```python
from build123d import *

# Parameters (mm, degrees)
BOSS_EXTRUDE1_DEPTH       = 3.5
SKETCH2_R                 = 9.5
CUT_EXTRUDE1_DEPTH        = 5
SKETCH3_R                 = 8.75
CUT_EXTRUDE2_DEPTH        = 59.736700622
SKETCH4_R                 = 9.5
CUT_EXTRUDE3_DEPTH        = 5
SKETCH5_R                 = 8.75
CUT_EXTRUDE4_DEPTH        = 59.736700622
SKETCH6_R                 = 17.5
SKETCH6_R_2               = 10
CUT_EXTRUDE5_DEPTH        = 0.5
SKETCH7_W                 = 1.5
SKETCH7_H                 = 1.5
FILLET1_START             = 2
FILLET1_DEPTH             = 2
MIRROR2_COPY_1_SKETCH_R   = 17.5
MIRROR2_COPY_1_SKETCH_R_2 = 10
MIRROR2_COPY_1_DEPTH      = 0.5
MIRROR2_COPY_2_SKETCH_W   = 1.5
MIRROR2_COPY_2_SKETCH_H   = 1.5
MIRROR2_START             = 2
MIRROR2_COPY_3_DEPTH      = 2


with BuildPart() as part:
    # Sketch1 → Boss-Extrude1 (new, symmetric)
    with BuildSketch(Plane(origin=(0, 0, 0), x_dir=(1, 0, 0), z_dir=(0, 1, 0))):
        with BuildLine():
            ThreePointArc((-21, 14.282856857), (-55, 0), (-21, -14.282856857))
            ThreePointArc((-21, -14.282856857), (0, -5.707142143), (21, -14.282856857))
            ThreePointArc((21, -14.282856857), (55, 0), (21, 14.282856857))
            ThreePointArc((21, 14.282856857), (0, 5.707142143), (-21, 14.282856857))
        make_face()
    extrude(amount=BOSS_EXTRUDE1_DEPTH, both=True)

    # Sketch2 → Cut-Extrude1 (cut)
    with BuildSketch(Plane(origin=(0, 3.5, 0), x_dir=(1, 0, 0), z_dir=(0, 1, 0))):
        with Locations(Location((-35, 0, 0), (0, 0, 270))):
            Circle(SKETCH2_R)
    extrude(amount=-CUT_EXTRUDE1_DEPTH, mode=Mode.SUBTRACT)

    # Sketch3 → Cut-Extrude2 (cut, through all)
    with BuildSketch(Plane(origin=(0, -1.5, 0), x_dir=(1, 0, 0), z_dir=(0, 1, 0))):
        with Locations(Location((-35, 0, 0), (0, 0, 270))):
            Circle(SKETCH3_R)
    extrude(amount=-CUT_EXTRUDE2_DEPTH, mode=Mode.SUBTRACT)

    # Sketch4 → Cut-Extrude3 (cut)
    with BuildSketch(Plane.XZ.offset(3.5)):
        with Locations(Location((35, 0, 0), (0, 0, 270))):
            Circle(SKETCH4_R)
    extrude(amount=-CUT_EXTRUDE3_DEPTH, mode=Mode.SUBTRACT)

    # Sketch5 → Cut-Extrude4 (cut, through all)
    with BuildSketch(Plane.XZ.offset(-1.5)):
        with Locations(Location((35, 0, 0), (0, 0, 270))):
            Circle(SKETCH5_R)
    extrude(amount=-CUT_EXTRUDE4_DEPTH, mode=Mode.SUBTRACT)

    # Sketch6 → Cut-Extrude5 (cut)
    with BuildSketch(Plane(origin=(0, 3.5, 0), x_dir=(1, 0, 0), z_dir=(0, 1, 0))):
        with Locations(Location((-35, 0, 0), (0, 0, 270))):
            Circle(SKETCH6_R)
        with Locations(Location((-35, 0, 0), (0, 0, 270))):
            Circle(SKETCH6_R_2, mode=Mode.SUBTRACT)
    cut_extrude5 = extrude(amount=-CUT_EXTRUDE5_DEPTH, mode=Mode.SUBTRACT)

    # Sketch7 → Cut-Revolve1 (revolve, cut)
    with BuildSketch(Plane.XY, mode=Mode.PRIVATE) as cut_revolve1_sk:
        with Locations((-54.25, 2.75)):
            Rectangle(SKETCH7_W, SKETCH7_H)
    cut_revolve1 = revolve(cut_revolve1_sk.sketch.rotate(Axis((-35, -6.63312042, 0), (0, 1, 0)), 270), axis=Axis((-35, -6.63312042, 0), (0, 1, 0)), mode=Mode.SUBTRACT)

    # Fillet1: read off the stored shape, not the designer's step
    # Fillet1 outline → Fillet1 (cut)
    with BuildSketch(Plane(origin=(0, 0, 0), x_dir=(1, 0, 0), z_dir=(0, 1, 0)).offset(FILLET1_START)):
        with BuildLine():
            ThreePointArc((-21, -14.282856857), (-17.348361604, -11.231963907), (-13.260269064, -8.796823223))
            ThreePointArc((-13.260269064, -8.796823223), (-15.460727643, -8.508452663), (-16.04026091, -6.366183602))
            ThreePointArc((-16.04026091, -6.366183602), (-18.051415131, -10.618167023), (-21, -14.282856857))
        make_face()
        with BuildLine():
            ThreePointArc((-21, 14.282856857), (-18.051415131, 10.618167023), (-16.04026091, 6.366183602))
            ThreePointArc((-16.04026091, 6.366183602), (-15.460727643, 8.508452663), (-13.260269064, 8.796823223))
            ThreePointArc((-13.260269064, 8.796823223), (-17.348361604, 11.231963907), (-21, 14.282856857))
        make_face()
    fillet1 = extrude(amount=FILLET1_DEPTH, mode=Mode.SUBTRACT)

    # Mirror1: Cut-Extrude5, Cut-Revolve1, Fillet1 across plane
    add(cut_extrude5.mirror(Plane.ZX), mode=Mode.SUBTRACT)
    add(cut_revolve1.mirror(Plane.ZX), mode=Mode.SUBTRACT)
    add(fillet1.mirror(Plane.ZX), mode=Mode.SUBTRACT)

    # Mirror2: Cut-Extrude5, Cut-Revolve1, Fillet1 across plane
    add(cut_extrude5.mirror(Plane(origin=(0, 0, 0), x_dir=(0, 0, 1), z_dir=(1, 0, 0))), mode=Mode.SUBTRACT)
    add(cut_revolve1.mirror(Plane(origin=(0, 0, 0), x_dir=(0, 0, 1), z_dir=(1, 0, 0))), mode=Mode.SUBTRACT)
    add(fillet1.mirror(Plane(origin=(0, 0, 0), x_dir=(0, 0, 1), z_dir=(1, 0, 0))), mode=Mode.SUBTRACT)

    # Mirror2 copy 1 sketch → Mirror2 copy 1 (cut)
    with BuildSketch(Plane(origin=(0, -3.5, 0), x_dir=(-1, 0, 0), z_dir=(0, -1, 0))):
        with Locations(Location((-35, 0, 0), (0, 0, 270))):
            Circle(MIRROR2_COPY_1_SKETCH_R)
        with Locations(Location((-35, 0, 0), (0, 0, 270))):
            Circle(MIRROR2_COPY_1_SKETCH_R_2, mode=Mode.SUBTRACT)
    extrude(amount=-MIRROR2_COPY_1_DEPTH, mode=Mode.SUBTRACT)

    # Mirror2 copy 2 sketch → Mirror2 copy 2 (revolve, cut)
    with BuildSketch(Plane(origin=(0, 0, 0), x_dir=(-1, 0, 0), z_dir=(0, 0, 1))):
        with Locations((-54.25, 2.75)):
            Rectangle(MIRROR2_COPY_2_SKETCH_W, MIRROR2_COPY_2_SKETCH_H)
    revolve(axis=Axis((35, 6.63312042, 0), (0, -1, 0)), mode=Mode.SUBTRACT)

    # Mirror2 copy 3 sketch → Mirror2 copy 3 (cut)
    with BuildSketch(Plane(origin=(0, 0, 0), x_dir=(-1, 0, 0), z_dir=(0, -1, 0)).offset(MIRROR2_START)):
        with BuildLine():
            ThreePointArc((-21, -14.282856857), (-17.348361604, -11.231963907), (-13.260269064, -8.796823223))
            ThreePointArc((-13.260269064, -8.796823223), (-15.460727643, -8.508452663), (-16.04026091, -6.366183602))
            ThreePointArc((-16.04026091, -6.366183602), (-18.051415131, -10.618167023), (-21, -14.282856857))
        make_face()
        with BuildLine():
            ThreePointArc((-21, 14.282856857), (-18.051415131, 10.618167023), (-16.04026091, 6.366183602))
            ThreePointArc((-16.04026091, 6.366183602), (-15.460727643, 8.508452663), (-13.260269064, 8.796823223))
            ThreePointArc((-13.260269064, 8.796823223), (-17.348361604, 11.231963907), (-21, 14.282856857))
        make_face()
    extrude(amount=MIRROR2_COPY_3_DEPTH, mode=Mode.SUBTRACT)


solid = part.part
```
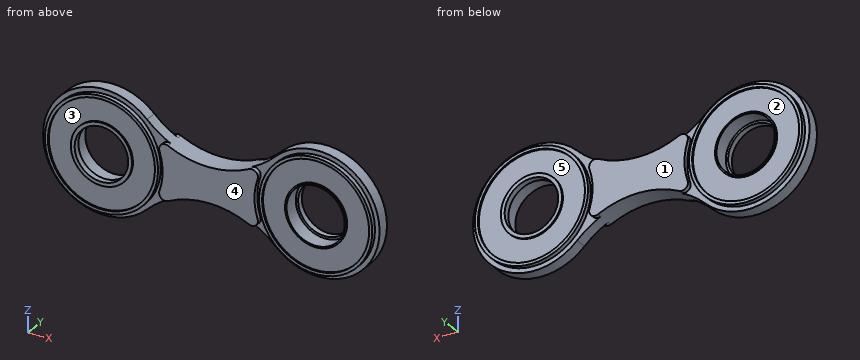
Design review of the part built by this model. Coordinates are the model's own, in mm. Face numbers are marked on the shaded views. A direction names the side the tool comes from. Give positions to 0.01 mm unless a question says otherwise; leave off trailing zeros. Write each loop counter-clockwise with the first axis right and the second up, starting at its lowest first coordinate (ties: lowest second). Pieces come first, ordered by that corner, then holes. Notation, with made-up numbers: (72, -10.5) - (79, -10.5) arc R27 ccw to (79, 7.5) - close; hole circle Ø11 at (40, 11). An arc over 180 degrees is marked (long way). Return JSON: item names as keys, results as strings. Group by question number.
(1) We need section D-D, the plane x = -5.5. Give the boundary of the cut face in (y, z).
(2) We need section A-A, the plane y = 0.25. Give the boundary of the cut face in (x, z), then the cut area to 3 significant figures.
(3) To check wall thickness, follow probe 1 along X at (y, z) = (-0.5, 0.5); probe 2 along X at (y, z) = (-1, 1); probe 3 along X at (y, z) = (-0.75, 8). State the ranges of each line that lie inside material, in increasing order.
(4) We need section C-C, the plane x = -46.5. Give the boundary of the cut face in (y, z), then the cut area to 3 significant figures.
(5) We need section B-B, the plane z = 0. Give the number of separate pieces and of enclosed holes in the cut face, then the cut area to 3 significant figures.
(6) Insertion check: pin 1 (4 mm diameter, centred on x = -20, z = -15, fed in from -Y); pin 2 (1 mm diameter, centred on y = 1, z = -11, fed in from -X); pin 3 (11.5 mm diameter, centred on x = 35, z = 0, fed in from -Y); pin 4 (3 mm diameter, centred on x = -39.5, z = 14.5, fed in from -Y). Each pin has a flat end and moves straight along its axis. Give the tip position at first contact, or say it passes through.
(7) Machinability: for the marked faces 1, 2 and 3, which of the approach directions +Z, -Z, +X, -X, +Y, -Y give a long, thin tool a straight path to every point of the face, cutting with its end or side? Answer none if there is none.
(8) Mouldability with a two-part tool opening along Z and no side actions: class the marked faces 4 and 5 as +Z half, -Z half, draft (parallel to the pull), parting line (faces both ways), or undercut.
Reported:
{
 "1": {"outline": "(-3.5, -6.22) - (3.5, -6.22) - (3.5, 6.22) - (-3.5, 6.22) - close"},
 "2": {"outline": "(-21, -14.28) arc R30 cw to (21, -14.28) arc R20 ccw (long way) to (21, 14.28) arc R30 cw to (-21, 14.28) arc R20 ccw (long way) to start; hole circle Ø19 at (-35, 0); hole circle Ø19 at (35, 0)", "area": "2,410 mm2"},
 "3": {"probe 1": "x = -54.99 to -44.49, -25.51 to 25.51, 44.49 to 54.99", "probe 2": "x = -54.97 to -44.45, -25.55 to 25.55, 44.45 to 54.97", "probe 3": "x = -53.33 to -40.12, -29.88 to -11.5, 11.5 to 29.88, 40.12 to 53.33"},
 "4": {"outline": "(-3.5, -14.49) - (-2, -14.49) - (-2, -16.36) - (2, -16.36) - (2, -14.49) - (3.5, -14.49) - (3.5, -13.19) - (3, -13.19) - (3, 13.19) - (3.5, 13.19) - (3.5, 14.49) - (2, 14.49) - (2, 16.36) - (-2, 16.36) - (-2, 14.49) - (-3.5, 14.49) - (-3.5, 13.19) - (-3, 13.19) - (-3, -13.19) - (-3.5, -13.19) - close", "area": "191 mm2"},
 "5": {"separate pieces": "3", "enclosed holes": "0", "area": "462 mm2"},
 "6": {"pin 1": "stops at y = -2", "pin 2": "stops at x = -52.02", "pin 3": "passes through", "pin 4": "stops at y = -3"},
 "7": {"face 1": "+Z, -Z, +X, -X, +Y", "face 2": "+Y", "face 3": "-Y"},
 "8": {"face 4": "draft", "face 5": "undercut"}
}
